Can you work these out from the drawing? Everything is in mm from the part's minimum corner. A direction names the side the tool comes from. Give positions to 0.01 mm unless a question says otherwise; leave off trailing zeros. Order: outer loops, then holes, each group sorted by start corner. A loop starts at its lowest first (then second) coordinate and runs counter-clockwise, first axis right, second up. Notation, with made-up numbers: M -32.75,20 L -9.75,20 A21 ccw -9.75,58 Z; hole C 15.5,72.25 d1. An arc over 180 degrees is marked long. Answer in a Markdown table with one row per item. Add a question column.
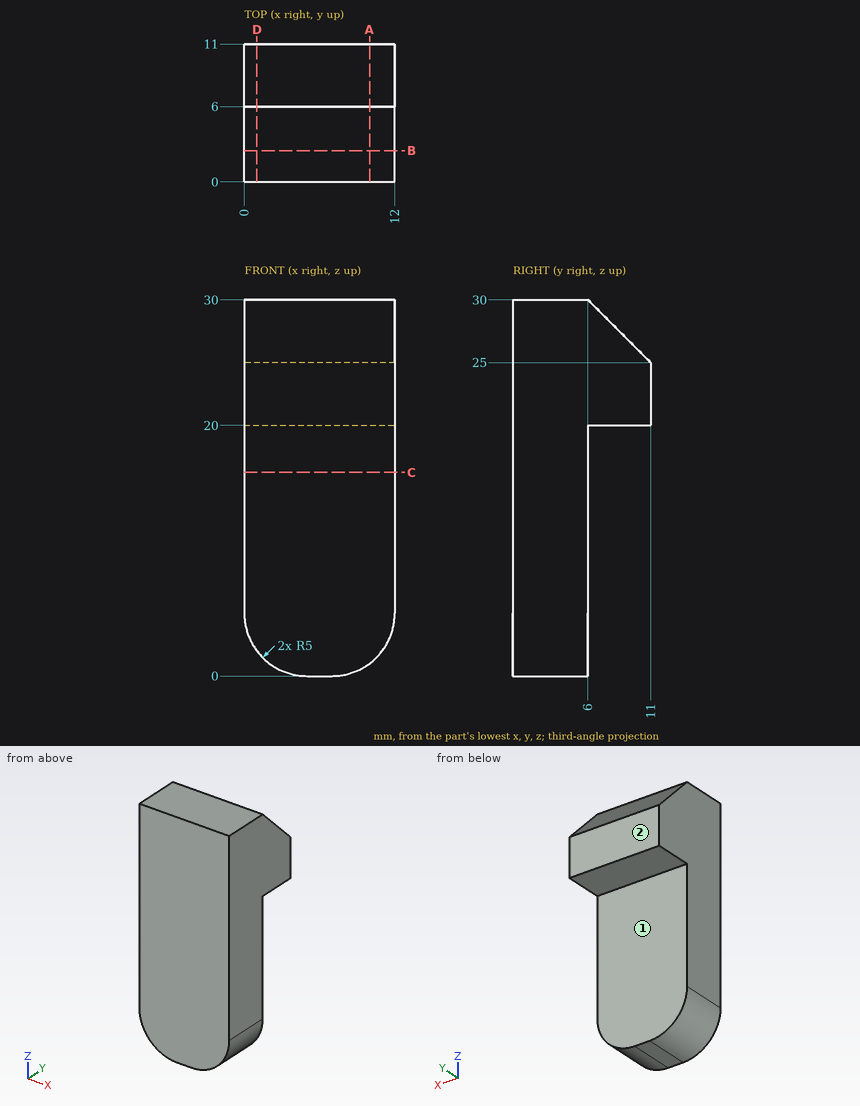
1. If I drill on line 1 along Y through (x, z) = (5.25, 9); line 2 along X through (y, z) = (1, 4.75); line 3 along Z through (x, y) = (3, 1.5), over which ranges is the centre line in solid material (lowest first)? Write a range as [from, to].
2. Suppose I cut it at B-B on y = 2.5. List the corners of the cut face in (x, z) for me.
3. Suppose I cut it at D-D on x = 1. List the corners of the cut face in (y, z) for me, plus the area to 4 significant figures.
4. For the marked faces 1 and 2, which set-ups out of +Z, -Z, +X, -X, +Y, -Y let a thin tool reach every point of the face, with its end or its side?
5. Will these pins go through, and if not, where does the flat tip stop? P1, Ø1, axis at y = 7.5, z = 4, coming from the +X side; P2, Ø6, axis at x = 9, z = 19.5, coming from the +Y side; P3, Ø2.5, axis at x = 3.5, y = 8.5, coming from the -Z side; P4, Ø1.5, axis at x = 2, y = 3, coming from the -Z side.
6. Suppose I cut it at A-A on x = 10. List the corners of the cut face in (y, z) for me, plus the area to 4 significant figures.
7. Suppose I cut it at C-C on z = 16.25. List the corners of the cut face in (x, y) for me, plus the area to 3 significant figures.
Findings below:
| question | item | result |
|---|---|---|
| 1 | line 1 | [0, 6] |
| 1 | line 2 | [0.01, 11.99] |
| 1 | line 3 | [0.42, 30] |
| 2 | outline | M 0,5 A5 ccw 5,0 L 7,0 A5 ccw 12,5 L 12,30 L 0,30 Z |
| 3 | outline | M 0,2 L 6,2 L 6,20 L 11,20 L 11,25 L 6,30 L 0,30 Z |
| 3 | area | 205.5 mm2 |
| 4 | face 1 | -Z, +X, -X, +Y |
| 4 | face 2 | +Z, -Z, +X, -X, +Y |
| 5 | P1 | through |
| 5 | P2 | y = 11 |
| 5 | P3 | z = 20 |
| 5 | P4 | z = 0.53 |
| 6 | outline | M 0,1 L 6,1 L 6,20 L 11,20 L 11,25 L 6,30 L 0,30 Z |
| 6 | area | 211.5 mm2 |
| 7 | outline | M 0,0 L 12,0 L 12,6 L 0,6 Z |
| 7 | area | 72.0 mm2 |
